from build123d import *

# Parameters (mm, degrees)
SKETCH2_R           = 76.2
BOSS_EXTRUDE1_DEPTH = 25.4
CUT_EXTRUDE1_DEPTH  = 76.2
CUT_EXTRUDE2_DEPTH  = 76.2
SKETCH8_W           = 5.08
SKETCH8_H           = 5.08
CUT_EXTRUDE4_DEPTH  = 50.8
CUT_EXTRUDE5_DEPTH  = 26.4
SKETCH10_R          = 2.159
CUT_EXTRUDE6_DEPTH  = 25.4


with BuildPart() as part:
    # Sketch2 → Boss-Extrude1 (new body)
    with BuildSketch(Plane.XY):
        Circle(SKETCH2_R)
    extrude(amount=BOSS_EXTRUDE1_DEPTH)

    # Sketch4 → Cut-Extrude1 (cut)
    with BuildSketch(Plane.XY.offset(25.4)):
        with BuildLine():
            Line((-75.519629236, 10.16), (75.519629236, 10.16))
            ThreePointArc((75.519629236, 10.16), (0, 76.2), (-75.519629236, 10.16))
        make_face()
    extrude(amount=-CUT_EXTRUDE1_DEPTH, mode=Mode.SUBTRACT)

    # Sketch5 → Cut-Extrude2 (cut)
    with BuildSketch(Plane.XY.offset(25.4)):
        with BuildLine():
            Line((49.396930897, 5.08), (-49.396930897, 5.08))
            Line((-49.396930897, 5.08), (-49.396930897, -51.166371944))
            ThreePointArc((-49.396930897, -51.166371944), (-41.049983197, -58.077132157), (-31.75, -63.639546667))
            Line((-31.75, -63.639546667), (31.75, -63.639546667))
            ThreePointArc((31.75, -63.639546667), (41.049983197, -58.077132157), (49.396930897, -51.166371944))
            Line((49.396930897, -51.166371944), (49.396930897, 5.08))
        make_face()
    extrude(amount=-CUT_EXTRUDE2_DEPTH, mode=Mode.SUBTRACT)

    # Sketch8 → Cut-Extrude4 (cut)
    with BuildSketch(Plane.XY.offset(25.4)):
        with Locations((0, -66.179546667)):
            Rectangle(SKETCH8_W, SKETCH8_H)
    extrude(amount=-CUT_EXTRUDE4_DEPTH, mode=Mode.SUBTRACT)

    # Sketch9 → Cut-Extrude5 (cut, through all)
    with BuildSketch(Plane.XY.offset(25.4)):
        with BuildLine():
            Line((54.476930897, 5.08), (76.030478099, 5.08))
            ThreePointArc((76.030478099, 5.08), (71.480790805, -26.399555791), (54.476930897, -53.279489487))
            Line((54.476930897, -53.279489487), (54.476930897, 5.08))
        make_face()
        with BuildLine():
            Line((-54.476930897, 5.08), (-54.476930897, -53.279489487))
            ThreePointArc((-54.476930897, -53.279489487), (-71.480790805, -26.399555791), (-76.030478099, 5.08))
            Line((-76.030478099, 5.08), (-54.476930897, 5.08))
        make_face()
    extrude(amount=-CUT_EXTRUDE5_DEPTH, mode=Mode.SUBTRACT)

    # Sketch10 → Cut-Extrude6 (cut)
    with BuildSketch(Plane(origin=(0, 10.16, 0), x_dir=(1, 0, 0), z_dir=(0, 1, 0))):
        with Locations((62.819629236, -12.7)):
            Circle(SKETCH10_R)
        with Locations((-62.819629236, -12.7)):
            Circle(SKETCH10_R)
    extrude(amount=-CUT_EXTRUDE6_DEPTH, mode=Mode.SUBTRACT)


solid = part.part
Input: part model. Units: mm. Frame: model coordinates. A direction names the side the tool comes from. Coordinates: 2 decimals unless noted, no trailing zeros. Order: outer loops, then holes, each group sorted by start corner. A loop starts at its lowest first (then second) coordinate and runs counter-clockwise, first axis right, second up. Notation, with made-up numbers: M 63.5,86.5 L 109.5,86.5 A16 ccw 109.5,92.5 Z; hole C 74,27.5 d9. An arc over 180 degrees is marked long. Write item = value, one per line. Start each with the question number.
(1) Section C-C on x = 36.5. Output: boundary loops of the cut face in (y, z), and give its area (3 significant figures).
(2) Reachability of faces 4 (the cylindrical face through (64.88, 7.66, 12.05)), 5 (the flat face through (1, 5.08, 13)), 6 (the flat face through (-54.477, -24, 13)), 7 (the flat face through (54.477, -25, 13)), 8 (the flat face through (-1, 10.16, 13)) from +Z, -Z, +X, -X, +Y, -Y: full face, straight path, thin tool, end or side. Return the list, or none.
(3) Section D-D on z = 20.25. Output: boundary loops of the cut face in (x, y), and give its area (3 significant figures).
(4) First-contact query: P1, Ø6, axis at y = -29, z = 3.5, coming from the +X side; P2, Ø3, axis at y = -17.5, z = 16, coming from the -X side; P3, Ø12, axis at x = 44, y = -20.5, coming from the +Z side; P4, Ø3, axis at x = 16, z = 9.5, coming from the -Y side. Flat tips, straight axial feed; report the tip coordinate or a pass-through.
(5) Pull-direction query (X, two-part tool) for faces 1 (the cylindrical face through (-0.85, -76.195, 12.522)), 2 (the flat face through (67, 5.08, 13)), 3 (the flat face through (-2.54, -66, 13)); classes: released by +X, released by -X, zero draft, split by the parting line, or undercut.
(6) Section A-A on y = -43.5. Output: boundary loops of the cut face in (x, z), and give its area (3 significant figures).
(7) Section B-B on z = 12.7. Output: boundary loops of the cut face in (x, y), and give its area (3 significant figures).
(8) Line query: line 1 along X through (y, z) = (-8, 17.75); line 2 along Y through (x, z) = (0, 21.25); line 3 along Y through (x, z) = (45, 17.5). Output: solid intervals per line, ascending. Write a range as [from, to].
Result set:
q1.outline = M -66.89,0 L -61.04,0 L -61.04,25.4 L -66.89,25.4 Z; M 5.08,0 L 10.16,0 L 10.16,25.4 L 5.08,25.4 Z
q1.area = 278 mm²
q2.face_4 = +Y, -Y
q2.face_5 = +Z, -Z
q2.face_6 = +Z, -Z, -X, -Y
q2.face_7 = +Z, -Z, +X, -Y
q2.face_8 = +Z, -Z, +X, -X, +Y
q3.outline = M -76.03,5.08 L -54.48,5.08 L -54.48,-53.28 A76.2 ccw 54.48,-53.28 L 54.48,5.08 L 76.03,5.08 A76.2 ccw 75.52,10.16 L -75.52,10.16 A76.2 ccw Z; hole M -49.4,-51.17 A71.12 ccw -31.75,-63.64 L -2.54,-63.64 L -2.54,-68.72 L 2.54,-68.72 L 2.54,-63.64 L 31.75,-63.64 A71.12 ccw 49.4,-51.17 L 49.4,5.08 L -49.4,5.08 Z
q3.area = 2,230 mm²
q4.P1 = 54.48
q4.P2 = -54.48
q4.P3 = 25.4
q4.P4 = -74.81
q5.face_1 = split by the parting line
q5.face_2 = zero draft
q5.face_3 = undercut
q6.outline = M -54.48,0 L -49.4,0 L -49.4,25.4 L -54.48,25.4 Z; M 49.4,0 L 54.48,0 L 54.48,25.4 L 49.4,25.4 Z
q6.area = 258 mm²
q7.outline = M -76.03,5.08 L -64.98,5.08 L -64.98,10.16 L -75.52,10.16 A76.2 ccw Z; M -60.66,5.08 L -54.48,5.08 L -54.48,-53.28 A76.2 ccw 54.48,-53.28 L 54.48,5.08 L 60.66,5.08 L 60.66,10.16 L -60.66,10.16 Z; M 64.98,5.08 L 76.03,5.08 A76.2 ccw 75.52,10.16 L 64.98,10.16 Z; hole M -49.4,-51.17 A71.12 ccw -31.75,-63.64 L -2.54,-63.64 L -2.54,-68.72 L 2.54,-68.72 L 2.54,-63.64 L 31.75,-63.64 A71.12 ccw 49.4,-51.17 L 49.4,5.08 L -49.4,5.08 Z
q7.area = 2,190 mm²
q8.line_1 = [-54.48, -49.4], [49.4, 54.48]
q8.line_2 = [-76.2, -68.72], [5.08, 10.16]
q8.line_3 = [-61.49, -55.07], [5.08, 10.16]
